Check sheet for the modelled part. Datum: model origin and axes. Units: mm. A direction names the side the tool comes from. Give positions to 0.01 mm unless a question says otherwise; leave off trailing zeros. Order: outer loops, then holes, each group sorted by start corner. A loop starts at its lowest first (then second) coordinate and runs counter-clockwise, first axis right, second up.
from build123d import *

# Parameters (mm, degrees)
SKETCH1_W           = 200
SKETCH1_H           = 100
BOSS_EXTRUDE1_DEPTH = 5
SKETCH2_W           = 200
SKETCH2_H           = 100
SKETCH2_W_2         = 190
SKETCH2_H_2         = 90
BOSS_EXTRUDE2_DEPTH = 70
SKETCH3_W           = 27
SKETCH3_H           = 40
CUT_EXTRUDE1_DEPTH  = 158.003184681
FILLET1_R           = 15


with BuildPart() as part:
    # Sketch1 → Boss-Extrude1 (new body)
    with BuildSketch(Plane(origin=(0, 0, 0), x_dir=(1, 0, 0), z_dir=(0, 1, 0))):
        Rectangle(SKETCH1_W, SKETCH1_H)
    extrude(amount=BOSS_EXTRUDE1_DEPTH)

    # Sketch2 → Boss-Extrude2 (add)
    with BuildSketch(Plane(origin=(0, 5, 0), x_dir=(1, 0, 0), z_dir=(0, 1, 0))):
        Rectangle(SKETCH2_W, SKETCH2_H)
        Rectangle(SKETCH2_W_2, SKETCH2_H_2, mode=Mode.SUBTRACT)
    extrude(amount=BOSS_EXTRUDE2_DEPTH)

    # Sketch3 → Cut-Extrude1 (cut, through all)
    with BuildSketch(Plane.XY.offset(-45)):
        with Locations((-81.5, 25)):
            Rectangle(SKETCH3_W, SKETCH3_H)
    extrude(amount=-CUT_EXTRUDE1_DEPTH, mode=Mode.SUBTRACT)

    # Fillet1
    # the kernel refuses this fillet: 15 mm, written as the material it adds along each edge
    with BuildSketch(Plane(origin=(95, 5, 45), x_dir=(0, 0, -1), z_dir=(0, 1, 0)), Plane(origin=(95, 5, -45), x_dir=(-1, 0, 0), z_dir=(0, 1, 0)), Plane(origin=(-95, 5, 45), x_dir=(1, 0, 0), z_dir=(0, 1, 0))) as fillet1_piece_1:
        with BuildLine():
            CenterArc((FILLET1_R, FILLET1_R), FILLET1_R, 180, 90)
            Line((0, FILLET1_R), (0, 0))
            Line((0, 0), (FILLET1_R, 0))
        make_face()
    extrude(amount=70)
    with BuildSketch(Plane(origin=(-95, 45, -45), x_dir=(1, 0, 0), z_dir=(0, 1, 0))) as fillet1_piece_2:
        with BuildLine():
            CenterArc((FILLET1_R, -FILLET1_R), FILLET1_R, 90, 90)
            Line((0, -FILLET1_R), (0, 0))
            Line((0, 0), (FILLET1_R, 0))
        make_face()
    extrude(amount=30)
    # the kernel refuses this fillet: 15 mm, written as the material it takes off along each edge
    with BuildSketch(Plane(origin=(100, 112.5, -50), x_dir=(-1, 0, 0), z_dir=(0, -1, 0)), Plane(origin=(-100, -37.5, -50), x_dir=(1, 0, 0), z_dir=(0, 1, 0)), Plane(origin=(100, 112.5, 50), x_dir=(0, 0, -1), z_dir=(0, -1, 0))) as fillet1_2_piece_1:
        with BuildLine():
            CenterArc((FILLET1_R, -FILLET1_R), FILLET1_R, 90, 90)
            Line((0, -FILLET1_R), (0, 0))
            Line((0, 0), (FILLET1_R, 0))
        make_face()
    extrude(amount=150, mode=Mode.SUBTRACT)
    with BuildSketch(Plane(origin=(-100, -37.5, 50), x_dir=(1, 0, 0), z_dir=(0, 1, 0))) as fillet1_2_piece_2:
        with BuildLine():
            CenterArc((FILLET1_R, FILLET1_R), FILLET1_R, 180, 90)
            Line((0, FILLET1_R), (0, 0))
            Line((0, 0), (FILLET1_R, 0))
        make_face()
    extrude(amount=150, mode=Mode.SUBTRACT)


solid = part.part
1) Section check D-D, the plane x = -21. Record the cut outline in (y, z).
Recorded:
outline: (0, -50) - (75, -50) - (75, -45) - (5, -45) - (5, 45) - (75, 45) - (75, 50) - (0, 50) - close
2) Section check C-C, the plane y = 33.5. Record the cut outline in (x, z).
Recorded:
outline: (-100, -35) arc R15 ccw to (-95, -46.18) - (-95, 30) arc R15 cw to (-80, 45) - (80, 45) arc R15 cw to (95, 30) - (95, -30) arc R15 cw to (80, -45) - (-68, -45) - (-68, -50) - (85, -50) arc R15 ccw to (100, -35) - (100, 35) arc R15 ccw to (85, 50) - (-85, 50) arc R15 ccw to (-100, 35) - close
3) Section check B-B, the plane x = -72.5. Record the cut outline in (y, z), then the cut area to 3 significant figures.
Recorded:
outline: (0, -50) - (5, -50) - (5, 45) - (75, 45) - (75, 50) - (0, 50) - close; (45, -50) - (75, -50) - (75, -45) - (45, -45) - close
area: 1,000 mm2
4) Section check A-A, the plane z = 19.5. Record the cut outline in (x, y).
Recorded:
outline: (-100, 0) - (100, 0) - (100, 75) - (95, 75) - (95, 5) - (-95, 5) - (-95, 75) - (-100, 75) - close
5) Set-up check for faces 4 (the face through (-1, 40, -45)), 5 (the face through (-83, 45, -46)), 6 (the face through (-95, 40, -8)): record each of +Z, -Z, +X, -X, +Y, -Y from which the full face is reachable in a straight line by a thin tool's end or side.
Recorded:
face 4: +Y
face 5: -Z
face 6: none
6) Draft check along X on faces 1 (the face through (95, 40, 0)), 2 (the face through (-1, 0, -1)), 3 (the face through (95.49, 38.03, -45.72)). Enter one of: +X half, -X half, draft (parallel to the pull), parting line (faces both ways), or undercut.
Recorded:
face 1: undercut
face 2: draft
face 3: +X half
7) Material ranges on L1, parallel to Z at x = 9, y = 44; L2, parallel to X at y = 33, z = 4; L3, parallel to Y at x = 45.5, z = -32, recorded low to high.
Recorded:
L1: z = -50 to -45, 45 to 50
L2: x = -100 to -95, 95 to 100
L3: y = 0 to 5
8) Depth check by flat-ended pin: pin 1 Ø10 at (x, z) = (56.5, -35) entering from +Y; pin 2 Ø4 at (y, z) = (16.5, -48.5) entering from -X. Enter the tip coordinate at first touch or a pass-through.
Recorded:
pin 1: stops at y = 5
pin 2: stops at x = -68
